Check sheet for the modelled part. Datum: model origin and axes. Units: mm. Give positions to 0.01 mm unless a question says otherwise; leave off trailing zeros. Write each loop counter-clockwise with the first axis right and the second up, starting at its lowest first coordinate (ties: lowest second). Pieces come first, ordered by that corner, then holes. Notation, with made-up numbers: (13, 38) -> (61, 38) arc R10 cw to (61, 49) -> close; hole circle Ø1 at (59, -10). An arc over 180 degrees is marked (long way). Use a Markdown table: item, result. Add a question column.
1. Cross-section at B-B (y = 429.5). Enter the section's corners in (x, z) (3 decimals), then the cut area to 3 significant figures.
2. Scan lines: probe 1 along X at (y, z) = (127.5, -1.5); probe 2 along Y at (x, z) = (-20, 1); probe 3 along Z at (x, y) = (3.5, 390). Record each from-to range of solid material in increasing order. Write a range as [from, to].
3. Gauge pin test, flat ends, axial feed: P1, Ø2, axis at y = 180, z = -8, coming from the +X side; P2, Ø4, axis at x = 11.5, z = -10, coming from the -Y side. Record the tip position at first contact, or that the pin passes through.
4. Cross-section at A-A (z = 0). Enter the section's corners in (x, y) (3 decimals), then the cut area to 3 significant figures.
5. Release check for a two-part mould opening along Y. For faces 1 (the flat face through (-8, 0, -5)), 2 (the flat face through (-7, 3.175, -7)), 3 (the cylindrical face through (-5.796, 264.576, -7.559)), 4 (the cylindrical face through (10.23, 1.57, 1.34)) record: released by +Y, released by -Y, zero draft, split by the parting line, or undercut.
from build123d import *

# Parameters (mm, degrees)
SKETCH1_R         = 9.525
SKETCH1_R_2       = 8.636
EXTRUDE1_DEPTH    = 546.1
EXTRUDE2_START    = -12.7
SKETCH2_R         = 34.671
SKETCH2_R_2       = 8.636
EXTRUDE2_DEPTH    = 12.7
SKETCH3_R         = 3.3655
EXTRUDE3_DEPTH    = 549.296786861
CIRPATTERN1_COUNT = 6
SKETCH4_R         = 10.31875
SKETCH4_R_2       = 8.636
EXTRUDE4_DEPTH    = 3.175


with BuildPart() as part:
    # Sketch1 → Extrude1 (new body)
    with BuildSketch(Plane(origin=(0, 0, 0), x_dir=(1, 0, 0), z_dir=(0, 1, 0))):
        with Locations(Location((0, 0, 0), (0, 0, 270))):
            Circle(SKETCH1_R)
        with Locations(Location((0, 0, 0), (0, 0, 270))):
            Circle(SKETCH1_R_2, mode=Mode.SUBTRACT)
    extrude(amount=EXTRUDE1_DEPTH)

    # Sketch2 → Extrude2 (add)
    with BuildSketch(Plane(origin=(0, 546.1, 0), x_dir=(1, 0, 0), z_dir=(0, 1, 0)).offset(EXTRUDE2_START)):
        with Locations(Location((0, 0, 0), (0, 0, 270))):
            Circle(SKETCH2_R)
        with Locations(Location((0, 0, 0), (0, 0, 270))):
            Circle(SKETCH2_R_2, mode=Mode.SUBTRACT)
    extrude(amount=EXTRUDE2_DEPTH)

    # Sketch3 → Extrude3 (cut, through all)
    with BuildSketch(Plane(origin=(0, 546.1, 0), x_dir=(1, 0, 0), z_dir=(0, 1, 0))):
        with Locations(Location((0, 29.3624, 0), (0, 0, 270))):
            Circle(SKETCH3_R)
    extrude3 = extrude(amount=-EXTRUDE3_DEPTH, mode=Mode.SUBTRACT)

    # CirPattern1: Extrude3 ×6 about axis
    cirpattern1_axis = Axis((0, 0, 0), (0, 1, 0))
    for i in range(1, CIRPATTERN1_COUNT):
        add(extrude3.rotate(cirpattern1_axis, i * 360 / CIRPATTERN1_COUNT), mode=Mode.SUBTRACT)

    # Sketch4 → Extrude4 (add)
    with BuildSketch(Plane.XZ):
        with Locations(Location((0, 0, 0), (0, 0, 270))):
            Circle(SKETCH4_R)
        with Locations(Location((0, 0, 0), (0, 0, 90))):
            Circle(SKETCH4_R_2, mode=Mode.SUBTRACT)
    extrude(amount=-EXTRUDE4_DEPTH)


solid = part.part
Worked answers:
| question | item | result |
|---|---|---|
| 1 | outline | circle Ø19.05 at (0, 0); hole circle Ø17.272 at (0, 0) |
| 1 | area | 50.7 mm² |
| 2 | probe 1 | x = [-9.41, -8.5], [8.5, 9.41] |
| 2 | probe 2 | y = [533.4, 546.1] |
| 2 | probe 3 | z = [-8.86, -7.89], [7.89, 8.86] |
| 3 | P1 | stops at x = 6.46 |
| 3 | P2 | stops at y = 533.4 |
| 4 | outline | (-34.671, 533.4) -> (-9.525, 533.4) -> (-9.525, 3.175) -> (-10.319, 3.175) -> (-10.319, 0) -> (-8.636, 0) -> (-8.636, 546.1) -> (-34.671, 546.1) -> close; (8.636, 0) -> (10.319, 0) -> (10.319, 3.175) -> (9.525, 3.175) -> (9.525, 533.4) -> (34.671, 533.4) -> (34.671, 546.1) -> (8.636, 546.1) -> close |
| 4 | area | 1,610 mm² |
| 5 | face 1 | released by -Y |
| 5 | face 2 | undercut |
| 5 | face 3 | undercut |
| 5 | face 4 | zero draft |
